```python
from build123d import *

# Parameters (mm, degrees)
SKETCH1_W           = 40
SKETCH1_H           = 10
BOSS_EXTRUDE1_DEPTH = 312.997959
SKETCH2_W           = 232.99
SKETCH2_H           = 1.2
CUT_EXTRUDE1_DEPTH  = 316.701951749
SKETCH3_R           = 1.9177
CUT_EXTRUDE2_DEPTH  = 316.701951749
CUT_EXTRUDE3_DEPTH  = 4.3
SKETCH5_R           = 2.762258299
CUT_EXTRUDE4_DEPTH  = 316.701951749
SKETCH6_W           = 4
SKETCH6_H           = 6.8326
CUT_EXTRUDE5_DEPTH  = 15
SKETCH7_W           = 232.5
SKETCH7_H           = 2.046306953
BOSS_EXTRUDE2_DEPTH = 60
CUT_EXTRUDE6_REACH  = 320.796
SKETCH8_W           = 215.9
SKETCH8_H           = 25
BOSS_EXTRUDE3_DEPTH = 3
SKETCH10_W          = 18
SKETCH10_H          = 4.844296322
BOSS_EXTRUDE4_DEPTH = 8.3
BOSS_EXTRUDE6_DEPTH = 232.745
FILLET1_R           = 0.7
SKETCH15_W          = 8.3
SKETCH15_H          = 18
BOSS_EXTRUDE8_DEPTH = 4.844296322
CUT_EXTRUDE8_DEPTH  = 319.961944969
CHAMFER1_SIZE       = 10.392304845
CHAMFER1_SIZE_2     = 6


with BuildPart() as part:
    # Sketch1 → Boss-Extrude1 (new body)
    with BuildSketch(Plane(origin=(0, 0, 0), x_dir=(0, 0, -1), z_dir=(1, 0, 0))):
        with Locations((20, 5)):
            Rectangle(SKETCH1_W, SKETCH1_H)
    extrude(amount=BOSS_EXTRUDE1_DEPTH)

    # Sketch2 → Cut-Extrude1 (cut, through all)
    with BuildSketch(Plane(origin=(0, 0, -40), x_dir=(-1, 0, 0), z_dir=(0, 0, -1))):
        with Locations((-156.4989795, 3.6)):
            Rectangle(SKETCH2_W, SKETCH2_H)
    extrude(amount=-CUT_EXTRUDE1_DEPTH, mode=Mode.SUBTRACT)

    # Sketch3 → Cut-Extrude2 (cut, through all)
    with BuildSketch(Plane(origin=(0, 10, 0), x_dir=(1, 0, 0), z_dir=(0, 1, 0))):
        with Locations(Location((294.997959, 25.5, 0), (0, 0, 270))):
            Circle(SKETCH3_R)
        with Locations(Location((294.997959, 14.5, 0), (0, 0, 270))):
            Circle(SKETCH3_R)
        with Locations(Location((18, 14.5, 0), (0, 0, 90))):
            Circle(SKETCH3_R)
        with Locations(Location((18, 25.5, 0), (0, 0, 90))):
            Circle(SKETCH3_R)
    extrude(amount=-CUT_EXTRUDE2_DEPTH, mode=Mode.SUBTRACT)

    # Sketch4 → Cut-Extrude3 (cut)
    with BuildSketch(Plane.XZ):
        Polygon((14.5837, -12.527598275), (14.5837, -16.472401725), (18, -18.444803449), (21.4163, -16.472401725), (21.4163, -12.527598275), (18, -10.555196551), align=None)
        Polygon((14.5837, -23.527598275), (14.5837, -27.472401725), (18, -29.444803449), (21.4163, -27.472401725), (21.4163, -23.527598275), (18, -21.555196551), align=None)
        Polygon((298.414259, -12.527598275), (294.997959, -10.555196551), (291.581659, -12.527598275), (291.581659, -16.472401725), (294.997959, -18.444803449), (298.414259, -16.472401725), align=None)
        Polygon((291.581659, -23.527598275), (291.581659, -27.472401725), (294.997959, -29.444803449), (298.414259, -27.472401725), (298.414259, -23.527598275), (294.997959, -21.555196551), align=None)
    extrude(amount=-CUT_EXTRUDE3_DEPTH, mode=Mode.SUBTRACT)

    # Sketch5 → Cut-Extrude4 (cut, through all)
    with BuildSketch(Plane.XY):
        with Locations((7, 5)):
            Circle(SKETCH5_R)
        with Locations(Location((305.997959, 5, 0), (0, 0, 180))):
            Circle(SKETCH5_R)
    extrude(amount=-CUT_EXTRUDE4_DEPTH, mode=Mode.SUBTRACT)

    # Sketch6 → Cut-Extrude5 (cut)
    with BuildSketch(Plane.ZY):
        with Locations((-31, 5)):
            Rectangle(SKETCH6_W, SKETCH6_H)
        with Locations((-9, 5)):
            Rectangle(SKETCH6_W, SKETCH6_H)
    extrude(amount=-CUT_EXTRUDE5_DEPTH, mode=Mode.SUBTRACT)

    # Sketch7 → Boss-Extrude2 (add)
    with BuildSketch(Plane.XY):
        with Locations((156.4989795, 1.023153477)):
            Rectangle(SKETCH7_W, SKETCH7_H)
    extrude(amount=BOSS_EXTRUDE2_DEPTH)

    # Sketch8 → Cut-Extrude6 (cut, up to next)
    with BuildSketch(Plane(origin=(0, 2.046306953, 0), x_dir=(1, 0, 0), z_dir=(0, 1, 0)), mode=Mode.PRIVATE) as cut_extrude6_sk1:
        with Locations((156.4989795, -47.5)):
            Rectangle(SKETCH8_W, SKETCH8_H)
    cut_extrude6_tool1 = extrude(cut_extrude6_sk1.sketch, amount=-CUT_EXTRUDE6_REACH, mode=Mode.PRIVATE) & part.part
    add(cut_extrude6_tool1.solids().sort_by_distance((156.49898, 2.046307, 47.5))[0], mode=Mode.SUBTRACT)

    # Sketch9 → Boss-Extrude3 (add)
    with BuildSketch(Plane.XZ):
        Polygon((0, -40), (0, 0), (40.2489795, 0), (40.2489795, 60), (48.5489795, 60), (48.5489795, 35), (264.4489795, 35), (264.4489795, 60), (272.7489795, 60), (272.7489795, 0), (312.997959, 0), (312.997959, -40), align=None)
        Polygon((17.997668231, -10.55519724), (14.582534712, -12.529617991), (14.584866481, -16.474420751), (18.002331769, -18.44480276), (21.417465288, -16.470382009), (21.415133519, -12.525579249), align=None, mode=Mode.SUBTRACT)
        Polygon((18.002331769, -21.55519724), (14.584866481, -23.525579249), (14.582534712, -27.470382009), (17.997668231, -29.44480276), (21.415133519, -27.474420751), (21.417465288, -23.529617991), align=None, mode=Mode.SUBTRACT)
        Polygon((295.000290769, -10.55519724), (291.582825481, -12.525579249), (291.580493712, -16.470382009), (294.995627231, -18.44480276), (298.413092519, -16.474420751), (298.415424288, -12.529617991), align=None, mode=Mode.SUBTRACT)
        Polygon((294.995627231, -21.55519724), (291.580493712, -23.529617991), (291.582825481, -27.474420751), (295.000290769, -29.44480276), (298.415424288, -27.470382009), (298.413092519, -23.525579249), align=None, mode=Mode.SUBTRACT)
    extrude(amount=BOSS_EXTRUDE3_DEPTH)

    # Sketch10 → Boss-Extrude4 (add)
    with BuildSketch(Plane.ZY.offset(-40.2489795)):
        with Locations((51, 4.468455114)):
            Rectangle(SKETCH10_W, SKETCH10_H)
    extrude(amount=-BOSS_EXTRUDE4_DEPTH)

    # Sketch12 → Boss-Extrude6 (add)
    with BuildSketch(Plane.ZY.offset(-40.2489795)):
        Polygon((0, 4.2), (7, 7.7), (0, 7.7), align=None)
    extrude(amount=-BOSS_EXTRUDE6_DEPTH)

    # Fillet1
    fillet1_edges = [part.edges().sort_by_distance(p)[0] for p in [
        (156.6214795, 7.7, 7),
    ]]
    fillet(fillet1_edges, radius=FILLET1_R)

    # Sketch15 → Boss-Extrude8 (add)
    with BuildSketch(Plane(origin=(0, 2.046306953, 0), x_dir=(1, 0, 0), z_dir=(0, 1, 0))):
        with Locations((268.5989795, -51)):
            Rectangle(SKETCH15_W, SKETCH15_H)
    extrude(amount=BOSS_EXTRUDE8_DEPTH)

    # Sketch16 → Cut-Extrude8 (cut, through all)
    with BuildSketch(Plane(origin=(0, 10, 0), x_dir=(1, 0, 0), z_dir=(0, 1, 0))):
        with BuildLine():
            Line((16.61580053, 24.172760339), (18, 22.729156574))
            Line((18, 22.729156574), (19.38419947, 24.172760339))
            ThreePointArc((19.38419947, 24.172760339), (18, 23.5823), (16.61580053, 24.172760339))
        make_face()
        with BuildLine():
            Line((16.61580053, 13.172760339), (18, 11.729156574))
            Line((18, 11.729156574), (19.38419947, 13.172760339))
            ThreePointArc((19.38419947, 13.172760339), (18, 12.5823), (16.61580053, 13.172760339))
        make_face()
        with BuildLine():
            Line((293.61375953, 13.172760339), (294.997959, 11.729156574))
            Line((294.997959, 11.729156574), (296.38215847, 13.172760339))
            ThreePointArc((296.38215847, 13.172760339), (294.997959, 12.5823), (293.61375953, 13.172760339))
        make_face()
        with BuildLine():
            Line((293.61375953, 24.172760339), (294.997959, 22.729156574))
            Line((294.997959, 22.729156574), (296.38215847, 24.172760339))
            ThreePointArc((296.38215847, 24.172760339), (294.997959, 23.5823), (293.61375953, 24.172760339))
        make_face()
    extrude(amount=-CUT_EXTRUDE8_DEPTH, mode=Mode.SUBTRACT)

    # Chamfer1
    # the kernel refuses this chamfer: 10.392304845, 6 mm, written as the material it takes off along each edge
    with BuildSketch(Plane(origin=(13.363195676, 6.890603275, 42), x_dir=(0, 0.019326765612700778, 0.9998132206222079), z_dir=(1, 0, 0))) as chamfer1_piece_1_section:
        Polygon((CHAMFER1_SIZE * 0.999813220662, CHAMFER1_SIZE * 0.0193267656135), (-CHAMFER1_SIZE_2 * 0.0193267656127, CHAMFER1_SIZE_2 * 0.999813220622), (0, 0), align=None)
    chamfer1_piece_1 = extrude(amount=62.071567647, mode=Mode.PRIVATE)
    chamfer1_piece_1 = split(chamfer1_piece_1, bisect_by=Plane(origin=(44.3989795, 2.046306953, 45.647661679), z_dir=(0, 1, 0)), keep=Keep.TOP, mode=Mode.PRIVATE)
    add(chamfer1_piece_1, mode=Mode.SUBTRACT)
    with BuildSketch(Plane(origin=(237.563195676, 6.890603275, 42), x_dir=(0, 0.019326765612700615, 0.9998132206222079), z_dir=(1, 0, 0))) as chamfer1_piece_2_section:
        Polygon((CHAMFER1_SIZE * 0.999813220662, CHAMFER1_SIZE * 0.0193267656135), (-CHAMFER1_SIZE_2 * 0.0193267656127, CHAMFER1_SIZE_2 * 0.999813220622), (0, 0), align=None)
    chamfer1_piece_2 = extrude(amount=62.071567647, mode=Mode.PRIVATE)
    chamfer1_piece_2 = split(chamfer1_piece_2, bisect_by=Plane(origin=(268.5989795, 2.046306953, 45.647661679), z_dir=(0, 1, 0)), keep=Keep.TOP, mode=Mode.PRIVATE)
    add(chamfer1_piece_2, mode=Mode.SUBTRACT)


solid = part.part
```
CAD build for the part. Positions are in the model's coordinates, mm. A direction names the side the tool comes from. Round coordinates to 2 decimals unless told otherwise and drop trailing zeros. Loops run counter-clockwise (first coordinate to the right, second up) from the corner with the lowest first, then second, coordinate; pieces in that order, holes last. Notation, with made-up numbers: M -34.5,6.25 L 8.5,6.25 A17 cw 8.5,38.25 Z; hole C 26,-40 d11. An arc over 180 degrees is marked long. Use a Markdown table: item, result. Add a question column.
(1) Cut at C-C (x = 118). Give the cut face in (y, z), and give its area (3 significant figures).
(2) Which spindle directions (+Z, -Z, +X, -X, +Y, -Y) get a long thin tool onto all of the face, cutting with end or side? Do faces 5 (the face through (159, 2, -40)), 6 (the face through (8.275, 2.549, -3.451)), 7 (the face through (48.549, 1, 50)), 8 (the face through (16, 4.3, -16)), 9 (the face through (9.1, 7.2, -33)). Say none if no direction does.
(3) Pull direction X, two halves, no side cores. Call faces 1 (the face through (9.1, 7.2, -7)), 2 (the face through (296.5, 4.3, -27.2)), 3 (the face through (0, 4, -20)), 4 (the face through (312.998, 4, -20)): +X half, -X half, draft (parallel to the pull), parting line (faces both ways), or undercut.
(4) Cut at D-D (z = 24.5). Give the cut face in (x, y).
(5) Drill centre lines: line 1 (Z direction, x = 18, y = 7.2); line 2 (X direction, y = 8.5, z = -14.5); line 3 (Y direction, x = 182, z = -13.5). Where is each one in solid material? Low to high.
(6) Cut at A-A (x = 7). Give the cut face in (y, z).
(7) Cut at B-B (z = -3). Give the cut face in (x, y).
(8) Flat gauge pins, fed straight in: pin 1 (3 mm diameter, centred on y = 6, z = 2, fed in from -X); pin 2 (5 mm diameter, centred on x = 117, z = 30.5, fed in from +Y). Where does each tip first touch, or does it go through?
Geometry says:
| question | item | result |
|---|---|---|
| 1 | outline | M -3,-40 L 3,-40 L 3,0 L 2.05,0 L 2.05,35 L -3,35 Z; M 4.2,-40 L 10,-40 L 10,0 L 7.7,0 L 7.7,4.03 A0.7 ccw 6.37,4.35 L 4.2,0 Z |
| 1 | area | 659 mm² |
| 2 | face 5 | -Z, +X, -X, +Y, -Y |
| 2 | face 6 | +Z, -Z |
| 2 | face 7 | +Z, +Y, -Y |
| 2 | face 8 | -Y |
| 2 | face 9 | -X |
| 3 | face 1 | draft |
| 3 | face 2 | undercut |
| 3 | face 3 | -X half |
| 3 | face 4 | +X half |
| 4 | outline | M 40.25,-3 L 272.75,-3 L 272.75,2.05 L 40.25,2.05 Z |
| 5 | line 1 | z = -40 to -27.42, -22.73 to -16.42, -11.73 to 0 |
| 5 | line 2 | x = 0 to 16.08, 19.92 to 293.08, 296.92 to 313 |
| 5 | line 3 | y = -3 to 3, 4.2 to 10 |
| 6 | outline | M -3,-40 L 2.24,-40 L 2.24,-33 L 1.58,-33 L 1.58,-29 L 2.24,-29 L 2.24,-11 L 1.58,-11 L 1.58,-7 L 2.24,-7 L 2.24,0 L -3,0 Z; M 7.76,-40 L 10,-40 L 10,0 L 7.76,0 L 7.76,-7 L 8.42,-7 L 8.42,-11 L 7.76,-11 L 7.76,-29 L 8.42,-29 L 8.42,-33 L 7.76,-33 Z |
| 7 | outline | M 0,-3 L 313,-3 L 313,10 L 0,10 Z; hole C 7,5 d5.52; hole M 40,3 L 272.99,3 L 272.99,4.2 L 40,4.2 Z; hole C 306,5 d5.52 |
| 8 | pin 1 | stops at x = 40.25 |
| 8 | pin 2 | stops at y = 2.05 |
